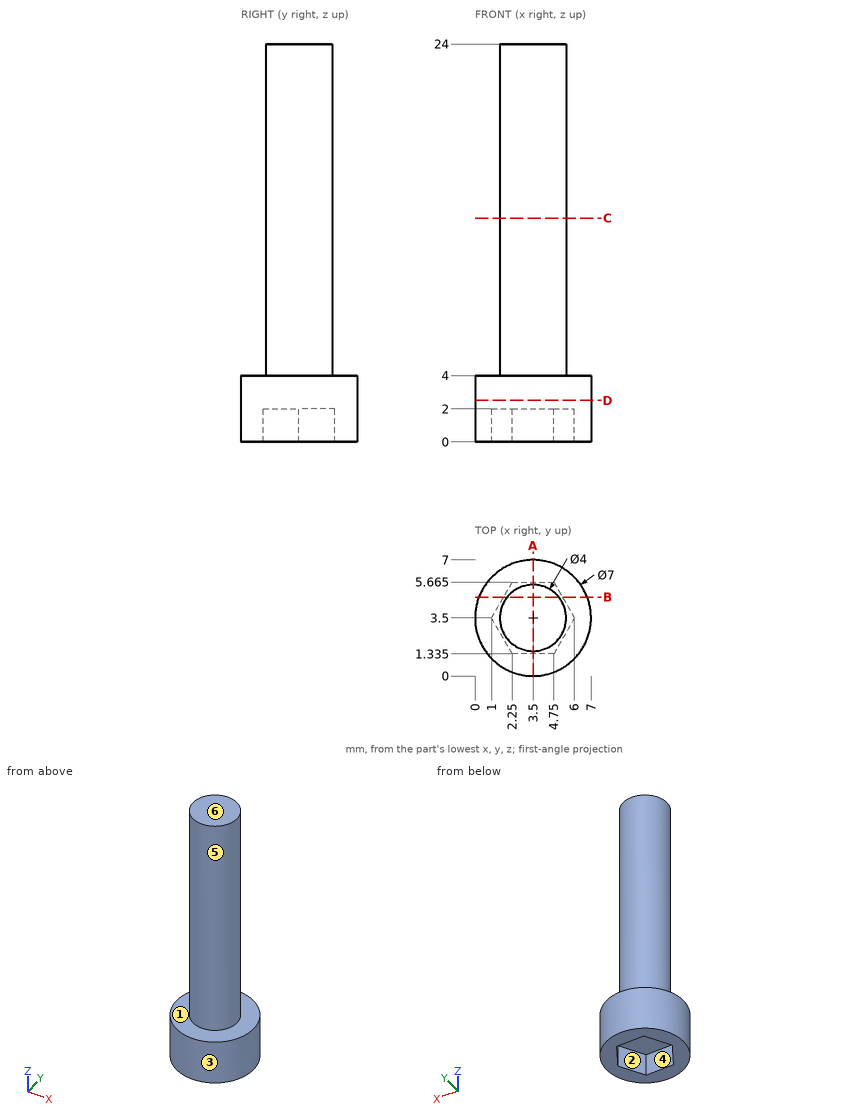
Print and shaded views of the part. All mm, measured from the part's lowest x, y and z. A direction names the side the tool comes from. Give positions to 0.01 mm unless a question says otherwise; leave off trailing zeros. Write each loop counter-clockwise with the first axis right and the second up, starting at its lowest first coordinate (ties: lowest second). Pieces come first, ordered by that corner, then holes. Notation, with made-up numbers: (67.25, 57) -> (71.25, 57) arc R13 ccw to (71.25, 76) -> close; hole circle Ø9 at (7, 39). An arc over 180 degrees is marked (long way). Use CSV: the item, a comma, the result in double quotes. Start each with the question number.
1) Cut at C-C on z = 13.5. List the corners of the cut face in (x, y).
2) Cut at D-D on z = 2.5. List the corners of the cut face in (x, y), plus the area to 3 significant figures.
3) Cut at B-B on y = 4.75. List the corners of the cut face in (x, z).
4) Two-plate mould, pull along X, no slides. Class the marked faces 1, 2 and 3: released by +X, released by -X, zero draft, split by the parting line, or undercut.
5) Tool access for the marked faces 4, 5 and 6: list every direction of +Z, -Z, +X, -X, +Y, -Y with a clear straight run to the whole face (end or side of a thin tool).
6) Drill centre lines: L1, parallel to Z at x = 6.25, y = 1.5; L2, parallel to Z at x = 3, y = 4.75; L3, parallel to Y at x = 5.5, z = 1. Where is each one in solid material? Low to high.
7) Cut at A-A on x = 3.5. List the corners of the cut face in (y, z) (3 decimals).
8) Pin check, flat tip, straight feed: P1, Ø3, axis at y = 5, z = 18.5, coming from the -X side. Stop position of the tip, or through.
Final values:
1,outline,"circle Ø4 at (3.5, 3.5)"
2,outline,"circle Ø7 at (3.5, 3.5)"
2,area,"38.5 mm2"
3,outline,"(0.23, 0) -> (1.72, 0) -> (1.72, 2) -> (5.28, 2) -> (5.28, 0) -> (6.77, 0) -> (6.77, 4) -> (5.06, 4) -> (5.06, 24) -> (1.94, 24) -> (1.94, 4) -> (0.23, 4) -> close"
4,face 1,"zero draft"
4,face 2,"undercut"
4,face 3,"split by the parting line"
5,face 4,"-Z"
5,face 5,"+Z"
5,face 6,"+Z, +X, -X, +Y, -Y"
6,L1,"z = 0 to 4"
6,L2,"z = 2 to 24"
6,L3,"y = 0.63 to 2.63, 4.37 to 6.37"
7,outline,"(0, 0) -> (1.335, 0) -> (1.335, 2) -> (5.665, 2) -> (5.665, 0) -> (7, 0) -> (7, 4) -> (5.5, 4) -> (5.5, 24) -> (1.5, 24) -> (1.5, 4) -> (0, 4) -> close"
8,P1,"stops at x = 1.5"
